Source: CAD feature listing. Evaluate the final solid. Frame: model axes, mm. Give positions to 0.01 mm unless a question says otherwise; leave off trailing zeros. Loops run counter-clockwise (first coordinate to the right, second up) from the corner with the lowest first, then second, coordinate; pieces in that order, holes last. Notation, with made-up numbers: (49.25, -5) -> (104.25, -5) arc R14 ccw to (104.25, 7) -> close; hole circle Ø2 at (71, -33.75). An arc over 180 degrees is marked (long way). Return JSON: item names as keys, results as strings. Group by question number.
```python
from build123d import *

# Parameters (mm, degrees)
F0_W     = 1000
F0_H     = 570
F0_R     = 25
F1_DEPTH = 25
F2_DEPTH = 25
F3_DEPTH = 25


with BuildPart() as f1:
    # F0 (on Top) → F1 (new body)
    with BuildSketch(Plane.XY):
        with Locations((-329.635155, -145.5779)):
            Rectangle(F0_W, F0_H)
        with Locations((-629.635155, -83.5779)):
            Circle(F0_R, mode=Mode.SUBTRACT)
        with Locations((-504.635155, -83.5779)):
            Circle(F0_R, mode=Mode.SUBTRACT)
        with Locations((-154.635155, -83.5779)):
            Circle(F0_R, mode=Mode.SUBTRACT)
        with Locations((-29.635155, -83.5779)):
            Circle(F0_R, mode=Mode.SUBTRACT)
    extrude(amount=F1_DEPTH)

    # F0 (on Top) → F2 (join)
    with BuildSketch(Plane.XY):
        with Locations((-329.635155, -145.5779)):
            Rectangle(F0_W, F0_H)
        with Locations((-629.635155, -83.5779)):
            Circle(F0_R, mode=Mode.SUBTRACT)
        with Locations((-504.635155, -83.5779)):
            Circle(F0_R, mode=Mode.SUBTRACT)
        with Locations((-154.635155, -83.5779)):
            Circle(F0_R, mode=Mode.SUBTRACT)
        with Locations((-29.635155, -83.5779)):
            Circle(F0_R, mode=Mode.SUBTRACT)
    extrude(amount=F2_DEPTH)

    # F0 (on Top) → F3 (join)
    with BuildSketch(Plane.XY):
        with Locations((-329.635155, -145.5779)):
            Rectangle(F0_W, F0_H)
        with Locations((-629.635155, -83.5779)):
            Circle(F0_R, mode=Mode.SUBTRACT)
        with Locations((-504.635155, -83.5779)):
            Circle(F0_R, mode=Mode.SUBTRACT)
        with Locations((-154.635155, -83.5779)):
            Circle(F0_R, mode=Mode.SUBTRACT)
        with Locations((-29.635155, -83.5779)):
            Circle(F0_R, mode=Mode.SUBTRACT)
    extrude(amount=F3_DEPTH)


solid = f1.part
```
1) Mould query, pull axis X, two halves, no side actions, for faces 1 (the face through (170.365, -150, 12)), 2 (the face through (-337, -142, 25)), 3 (the face through (-179.61, -82.48, 12.32)). Classes: released by +X, released by -X, zero draft, split by the parting line, or undercut.
2) Cut plane B-B on x = -27.5. Return loops of the section in (y, z).
3) Cut plane A-A on x = -148. Return loops of the section in (y, z), then the cut area to 3 significant figures.
4) Material intervals for line 1 (Y direction, x = -147.5, z = 6.5); line 2 (X direction, y = -100, z = 11.5); line 3 (Y direction, x = -37, z = 5.5), sorted ascending.
Calculated:
{
 "1": {"face 1": "released by +X", "face 2": "zero draft", "face 3": "undercut"},
 "2": {"outline": "(-430.58, 0) -> (-108.49, 0) -> (-108.49, 25) -> (-430.58, 25) -> close; (-58.67, 0) -> (139.42, 0) -> (139.42, 25) -> (-58.67, 25) -> close"},
 "3": {"outline": "(-430.58, 0) -> (-107.68, 0) -> (-107.68, 25) -> (-430.58, 25) -> close; (-59.47, 0) -> (139.42, 0) -> (139.42, 25) -> (-59.47, 25) -> close", "area": "13,000 mm2"},
 "4": {"line 1": "-430.58 to -107.54, -59.62 to 139.42", "line 2": "-829.64 to -648.48, -610.79 to -523.48, -485.79 to -173.48, -135.79 to -48.48, -10.79 to 170.36", "line 3": "-430.58 to -107.47, -59.69 to 139.42"}
}
